The model under review builds one solid part; all positions refer to its coordinate system, in mm. A direction names the side the tool comes from. Coordinates: 2 decimals unless noted, no trailing zeros. Order: outer loops, then holes, each group sorted by start corner. A loop starts at its lowest first (then second) coordinate and runs counter-clockwise, first axis right, second up.
from build123d import *

# Parameters (mm, degrees)
SKETCH_R      = 1.65
SKETCH_R_2    = 1.9
PAD_DEPTH     = 3
SKETCH001_R   = 3.5
SKETCH001_R_2 = 1.9
PAD001_DEPTH  = 3.5
CHAMFER_SIZE  = 0.4


with BuildPart() as part:
    # Sketch → Pad (new body)
    with BuildSketch(Plane.XY):
        Polygon((-1, -13), (1, -13), (13, -1), (13, 1), (7, 7), (-4, 7), (-7, 4), (-7, -7), align=None)
        with Locations((0, -10)):
            Circle(SKETCH_R, mode=Mode.SUBTRACT)
        with Locations((10, 0)):
            Circle(SKETCH_R, mode=Mode.SUBTRACT)
        with Locations((-3, 3)):
            Circle(SKETCH_R_2, mode=Mode.SUBTRACT)
    extrude(amount=PAD_DEPTH)

    # Sketch001 (on Face13 of Pad) → Pad001 (join)
    with BuildSketch(Plane.XY.offset(3)):
        with Locations((-3, 3)):
            Circle(SKETCH001_R)
        with Locations((-3, 3)):
            Circle(SKETCH001_R_2, mode=Mode.SUBTRACT)
    extrude(amount=PAD001_DEPTH)

    # Chamfer
    chamfer_edges = [part.edges().sort_by_distance(p)[0] for p in [
        (-4.9, 3, 0),
    ]]
    chamfer(chamfer_edges, length=CHAMFER_SIZE)


solid = part.part
(1) Consider section B-B (y = -10). Give the boundary of the cut face in (x, z), then the cut area to 3 significant figures.
(2) Consider section C-C (z = 2.5). Give the boundary of the cut face in (x, y), then the cut area to 3 significant figures.
(3) Wall thickness on line 1 (Y direction, x = 0, z = 1.65); line 2 (X direction, y = 1.5, z = 1); line 3 (Y direction, x = -3, z = 4): over which ranges is each line inside the solid? List them lowest first.
(4) The part is to be moulded in two halves that separate along Y. For faces 3 (the face through (0, -13, 1)), 4 (the face through (11.524, -0.632, 1.479)), 5 (the face through (3, -3, 3)), say which applies: +Y half, -Y half, draft (parallel to the pull), parting line (faces both ways), or undercut.
(5) Insertion check: pin 1 Ø2 at (x, y) = (6, 4) entering from +Z; pin 2 Ø3 at (x, y) = (0, -10) entering from +Z; pin 3 Ø1.5 at (y, z) = (3.5, 5.5) entering from +X. Each pin has a flat end and moves straight along its axis. Give the tip position at first contact, or say it passes through.
(6) Tool access review of faces 1 (the face through (0.34, 4.05, 4.73)), 2 (the face through (-1.188, 3.571, 3.407)): name each direction out of +Z, -Z, +X, -X, +Y, -Y from which nothing blocks a thin tool from reaching the whole face with its end or side.
(7) Consider section A-A (x = -3). Give the boundary of the cut face in (y, z), then the cut area to 3 significant figures.
Findings:
1. outline: (-4, 0) - (-1.65, 0) - (-1.65, 3) - (-4, 3) - close; (1.65, 0) - (4, 0) - (4, 3) - (1.65, 3) - close
1. area: 14.1 mm2
2. outline: (-7, -7) - (-1, -13) - (1, -13) - (13, -1) - (13, 1) - (7, 7) - (-4, 7) - (-7, 4) - close; hole circle Ø3.8 at (-3, 3); hole circle Ø3.3 at (0, -10); hole circle Ø3.3 at (10, 0)
2. area: 259 mm2
3. line 1: y = -13 to -11.65, -8.35 to 7
3. line 2: x = -7 to -4.17, -1.83 to 9.31, 10.69 to 12.5
3. line 3: y = -0.5 to 1.1, 4.9 to 6.5
4. face 3: -Y half
4. face 4: undercut
4. face 5: draft
5. pin 1: stops at z = 3
5. pin 2: passes through
5. pin 3: stops at x = 0.5
6. face 1: +Z
6. face 2: +Z, -Z
7. outline: (-11, 0) - (0.7, 0) - (1.1, 0.4) - (1.1, 6.5) - (-0.5, 6.5) - (-0.5, 3) - (-11, 3) - close; (4.9, 0.4) - (5.3, 0) - (7, 0) - (7, 3) - (6.5, 3) - (6.5, 6.5) - (4.9, 6.5) - close
7. area: 53.6 mm2
